Geometry check sheet. Reference: drawing and pictorial views, mm from the part's lowest x, y, z. Give positions to 0.01 mm unless a question says otherwise; leave off trailing zeros. Loops run counter-clockwise (first coordinate to the right, second up) from the corner with the lowest first, then second, coordinate; pieces in that order, holes last. Notation, with made-up numbers: (80.5, -16.75) -> (131.5, -16.75) arc R4 ccw to (131.5, -10.75) -> close; hole circle Ø10 at (25.5, -12.75). An arc over 180 degrees is marked (long way). One line per item, written item: value. Start each with the question number.
(1) Sectioned sample at D-D, the plane x = 111.5. Record the cut outline in (y, z) (1 decimal).
(2) Sectioned sample at C-C, the plane x = 202.5. Record the cut outline in (y, z), then the cut area to 3 significant figures.
(3) Sectioned sample at B-B, the plane x = 140. Record the cut outline in (y, z).
(4) Draft check along Z on the marked faces 1 and 2. Enter one of: pulls with the +Z half, pulls with the -Z half, needs draft (parallel to the pull), parting line crosses it, or undercut.
(5) Scan lines: line 1 along Z through (x, y) = (140, 2.4); line 2 along Z through (x, y) = (210, 3.35); line 3 along Z through (x, y) = (197.5, 3.3) (1 decimal). Record each from-to range of solid material in increasing order. Write a range as from..to.
(6) Sectioned sample at A-A, the plane x = 40. Record the cut outline in (y, z).
(7) Gauge pin test, flat ends, axial feed: pin 1 Ø3 at (x, z) = (97, 102) entering from +Y; pin 2 Ø3.5 at (x, z) = (198, 92.78) entering from +Y. Record the tip position at first contact, or that the pin passes through.
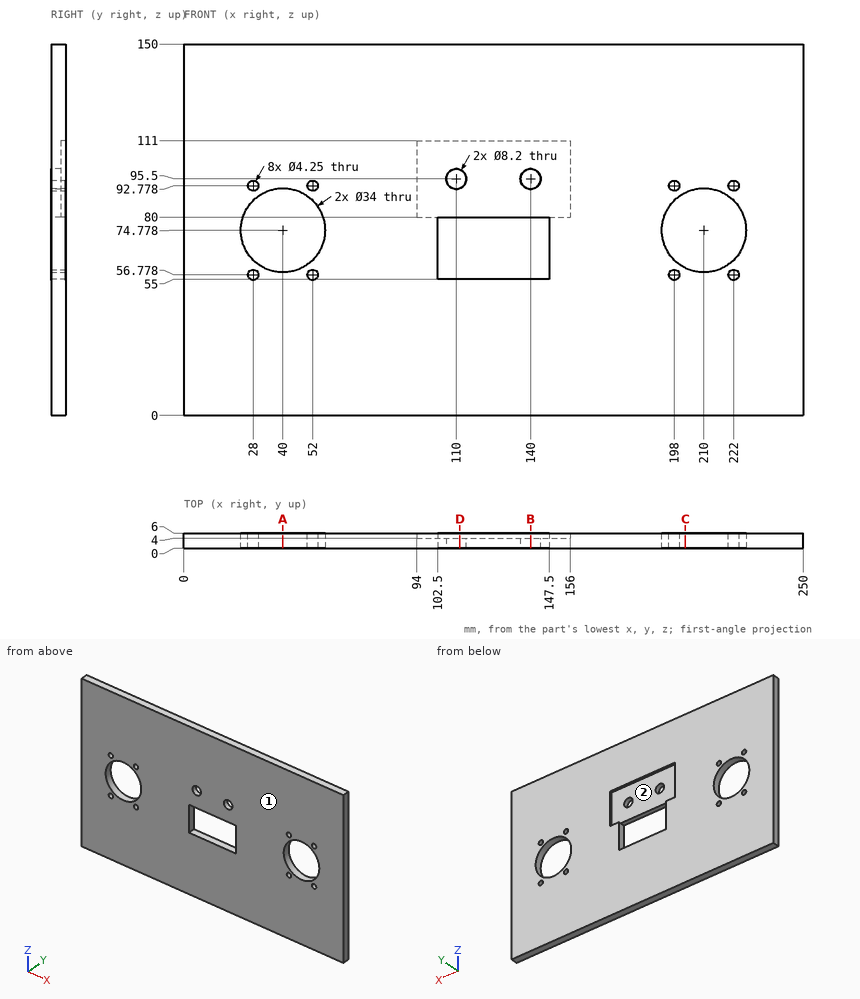
Calculated:
1. outline: (0, 0) -> (6, 0) -> (6, 55) -> (0, 55) -> close; (0, 80) -> (4, 80) -> (4, 91.7) -> (0, 91.7) -> close; (0, 99.3) -> (4, 99.3) -> (4, 111) -> (6, 111) -> (6, 150) -> (0, 150) -> close
2. outline: (0, 0) -> (6, 0) -> (6, 59.52) -> (0, 59.52) -> close; (0, 90.03) -> (6, 90.03) -> (6, 150) -> (0, 150) -> close
2. area: 717 mm2
3. outline: (0, 0) -> (6, 0) -> (6, 55) -> (0, 55) -> close; (0, 80) -> (4, 80) -> (4, 91.4) -> (0, 91.4) -> close; (0, 99.6) -> (4, 99.6) -> (4, 111) -> (6, 111) -> (6, 150) -> (0, 150) -> close
4. face 1: needs draft
4. face 2: undercut
5. line 1: z = 0..55, 80..91.4, 99.6..150
5. line 2: z = 0..57.78, 91.78..150
5. line 3: z = 0..54.7, 58.8..63.3, 86.3..90.7, 94.8..150
6. outline: (0, 0) -> (6, 0) -> (6, 57.78) -> (0, 57.78) -> close; (0, 91.78) -> (6, 91.78) -> (6, 150) -> (0, 150) -> close
7. pin 1: stops at y = 4
7. pin 2: passes through
